Source: three-view drawing plus pictorial views. Frame: mm from the lowest corner of the part. A direction names the side the tool comes from. Round coordinates to 2 decimals unless told otherwise and drop trailing zeros. Order: outer loops, then holes, each group sorted by start corner. A loop starts at its lowest first (then second) coordinate and runs counter-clockwise, first axis right, second up. Notation, with made-up numbers: (81, -33.75) -> (95, -33.75) arc R20 ccw to (95, -14.75) -> close; hole circle Ø3 at (29, 61.5). An arc over 180 degrees is marked (long way). Answer as CSV lines item,"result". Start each with the question number.
1) First-contact query: P1, Ø3, axis at x = 25.5, y = 7, coming from the -Z side; P2, Ø2, axis at x = 11.5, z = 4.5, coming from the -Y side. Flat tips, straight axial feed; report the tip coordinate or a pass-through.
2) Access query for the marked faces 1, 2, 3 and 4. Directions: +Z, -Z, +X, -X, +Y, -Y. A direction counts if a zero-diameter tool reaches every point of the face in a straight line with its end or side. Return the directions, or none.
3) Line query: L1, parallel to Z at x = 5, y = 16.25; L2, parallel to X at y = 11.75, z = 3; L3, parallel to X at y = 19, z = 4.5. Output: solid intervals per line, ascending.
4) Mould query, pull axis Z, two halves, no side actions, for the marked faces 5, 6 and 7. Classes: +Z half, -Z half, draft (parallel to the pull), parting line (faces both ways), or undercut.
5) Section query C-C, the plane z = 9.25. Output: boundary loops of the cut face in (x, y).
6) Section query A-A, the plane x = 45. Output: boundary loops of the cut face in (y, z), and give its area (3 significant figures).
7) Section query D-D, the plane x = 13. Output: boundary loops of the cut face in (y, z).
8) Section query B-B, the plane y = 8.5. Output: boundary loops of the cut face in (x, z), and give its area (3 significant figures).
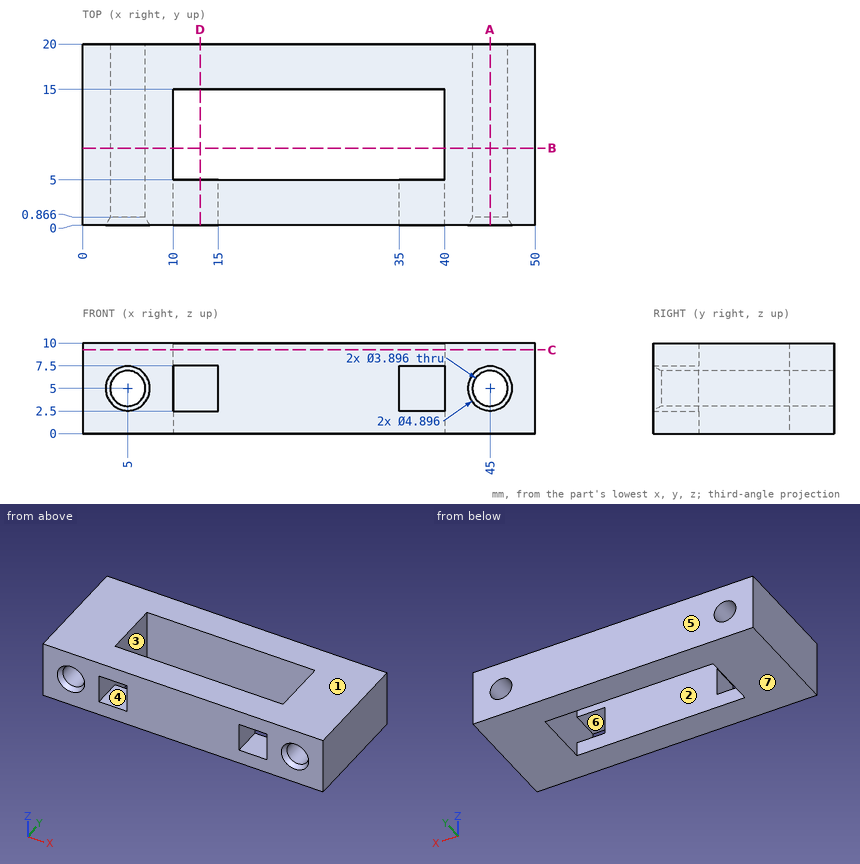
Findings:
1,P1,"passes through"
1,P2,"stops at y = 15"
2,face 1,"+Z, +X, -X, +Y, -Y"
2,face 2,"+Z, -Z"
2,face 3,"none"
2,face 4,"-Y"
3,L1,"z = 0 to 3.05, 6.95 to 10"
3,L2,"x = 0 to 10, 40 to 50"
3,L3,"x = 0 to 3.12, 6.88 to 43.12, 46.88 to 50"
4,face 5,"draft"
4,face 6,"undercut"
4,face 7,"-Z half"
5,outline,"(0, 0) -> (50, 0) -> (50, 20) -> (0, 20) -> close; hole (10, 5) -> (40, 5) -> (40, 15) -> (10, 15) -> close"
6,outline,"(0, 0) -> (20, 0) -> (20, 3.05) -> (0.87, 3.05) -> (0, 2.55) -> close; (0, 7.45) -> (0.87, 6.95) -> (20, 6.95) -> (20, 10) -> (0, 10) -> close"
6,area,"122 mm^2"
7,outline,"(0, 0) -> (5, 0) -> (5, 2.5) -> (0, 2.5) -> close; (0, 7.5) -> (5, 7.5) -> (5, 10) -> (0, 10) -> close; (15, 0) -> (20, 0) -> (20, 10) -> (15, 10) -> close"
8,outline,"(0, 0) -> (10, 0) -> (10, 10) -> (0, 10) -> close; (40, 0) -> (50, 0) -> (50, 10) -> (40, 10) -> close; hole circle Ø3.9 at (5, 5); hole circle Ø3.9 at (45, 5)"
8,area,"176 mm^2"
